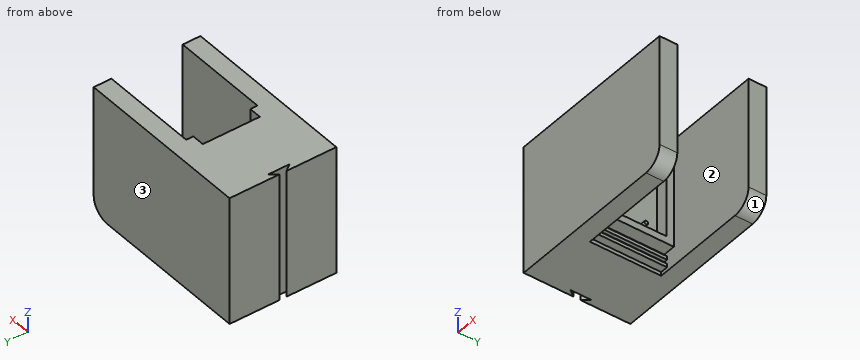
```python
from build123d import *

# Parameters (mm, degrees)
PAD_DEPTH       = 40.15
SKETCH001_W     = 72.15
SKETCH001_H     = 10
PAD001_DEPTH    = 100
FILLET_R        = 10
SKETCH002_W     = 57.4
SKETCH002_H     = 32.15
POCKET_DEPTH    = 7
SKETCH003_R     = 1.05
PAD002_DEPTH    = 3
POCKET001_DEPTH = 72.151


with BuildPart() as part:
    # Sketch → Pad (new body)
    with BuildSketch(Plane(origin=(24.695071, 0, 0), x_dir=(0, 0, 1), z_dir=(0, 1, 0))):
        Polygon((-27.089598, 5.251773), (34.310402, 5.251773), (34.310402, -39.748227), (-37.839598, -39.748227), (-37.839598, -4.048227), (-35.689598, -4.048227), (-35.689598, 0.251773), (-33.689598, 0.251773), (-33.689598, -1.748227), (-31.389598, -1.748227), (-31.389598, 0.251773), (-29.389598, 0.251773), (-29.389598, -1.748227), (-27.089598, -1.748227), align=None)
    extrude(amount=PAD_DEPTH)

    # Sketch001 (on Face4 of Pad) → Pad001 (join)
    with BuildSketch(Plane.ZY.offset(15.053156)):
        with Locations((-1.764598, -5)):
            Rectangle(SKETCH001_W, SKETCH001_H)
        with Locations((-1.764598, 45.15)):
            Rectangle(SKETCH001_W, SKETCH001_H)
    extrude(amount=-PAD001_DEPTH)

    # Fillet
    fillet_edges = [part.edges().sort_by_distance(p)[0] for p in [
        (84.946844, -5, -37.839598),
        (84.946844, 45.15, -37.839598),
    ]]
    fillet(fillet_edges, radius=FILLET_R)

    # Sketch002 (on Face6 of Fillet) → Pocket (cut)
    with BuildSketch(Plane(origin=(29.946844, 0, 0), x_dir=(0, 0, -1), z_dir=(1, 0, 0))):
        with Locations((-5.610402, 20.075)):
            Rectangle(SKETCH002_W, SKETCH002_H)
    extrude(amount=-POCKET_DEPTH, mode=Mode.SUBTRACT)

    # Sketch003 (on Face25 of Pocket) → Pad002 (join)
    with BuildSketch(Plane(origin=(22.946844, 0, 0), x_dir=(0, 0, -1), z_dir=(1, 0, 0))):
        with Locations((16.789598, 11.183873)):
            Circle(SKETCH003_R)
        with Locations((16.789598, 27.683873)):
            Circle(SKETCH003_R)
        with Locations((-7.210402, 11.183873)):
            Circle(SKETCH003_R)
    extrude(amount=PAD002_DEPTH)

    # Sketch004 (on Face20 of Pad002) → Pocket001 (cut, through all)
    with BuildSketch(Plane(origin=(24.695071, 0, -37.839598), x_dir=(-1, 0, 0), z_dir=(0, 0, -1))):
        Polygon((36.748227, 26.075), (39.748227, 22.075), (39.748227, 18.075), (36.748227, 14.075), align=None)
    extrude(amount=-POCKET001_DEPTH, mode=Mode.SUBTRACT)


solid = part.part
```
Verification items for the finished model (mm, model axes). Face numbers are marked on the shaded views. Coordinates: 2 decimals unless noted, no trailing zeros. Order: outer loops, then holes, each group sorted by start corner. A loop starts at its lowest first (then second) coordinate and runs counter-clockwise, first axis right, second up. Notation, with made-up numbers: (-6.5, 14) - (43.5, 14) arc R9 cw to (43.5, 20) - close; hole circle Ø3 at (88.5, 54). An arc over 180 degrees is marked (long way). Return JSON: item names as keys, results as strings.
(1) Section check A-A, the plane x = 42.5. Record the cut outline in (y, z).
Filled sheet:
{"outline": "(-10, -37.84) - (0, -37.84) - (0, 34.31) - (-10, 34.31) - close; (40.15, -37.84) - (50.15, -37.84) - (50.15, 34.31) - (40.15, 34.31) - close"}
(2) Mould release check, pull along Y, two halves, no side actions. Record for the marked faces 1, 2 and 3: pulls with the +Y half, pulls with the -Y half, needs draft (parallel to the pull), parting line crosses it, or undercut.
Filled sheet:
{"face 1": "needs draft", "face 2": "undercut", "face 3": "pulls with the +Y half"}
(3) Go/stop test with flat-tipped pins: pin 1 (5 mm diameter, centred on y = 34.5, z = 11.5, fed in from +X); pin 2 (1 mm diameter, centred on y = 18, z = -30.5, fed in from +X); pin 3 (5 mm diameter, centred on x = 33.5, y = 19.5, fed in from +Z); pin 4 (2.5 mm diameter, centred on y = 11.5, z = -37, fed in from +X). Record where each tip stops, or that it passes through.
Filled sheet:
{"pin 1": "stops at x = 29.95", "pin 2": "stops at x = 24.95", "pin 3": "passes through", "pin 4": "stops at x = 20.65"}
(4) Section check B-B, the plane z = -2.5. Record the cut outline in (x, y) (3 decimals).
Filled sheet:
{"outline": "(-15.053, -10) - (84.947, -10) - (84.947, 0) - (29.947, 0) - (29.947, 4) - (22.947, 4) - (22.947, 36.15) - (29.947, 36.15) - (29.947, 40.15) - (84.947, 40.15) - (84.947, 50.15) - (-15.053, 50.15) - (-15.053, 22.075) - (-12.053, 26.075) - (-12.053, 14.075) - (-15.053, 18.075) - close"}
(5) Section check C-C, the plane y = 8.5. Record the cut outline in (x, z).
Filled sheet:
{"outline": "(-15.05, -37.84) - (20.65, -37.84) - (20.65, -35.69) - (24.95, -35.69) - (24.95, -33.69) - (22.95, -33.69) - (22.95, -31.39) - (24.95, -31.39) - (24.95, -29.39) - (22.95, -29.39) - (22.95, -27.09) - (29.95, -27.09) - (29.95, -23.09) - (22.95, -23.09) - (22.95, 34.31) - (-15.05, 34.31) - close"}
(6) Thickness scan on line 1 along Y through (x, z) = (34, 4.5); line 2 along Y through (x, z) = (29.5, 9.5); line 3 along X through (y, z) = (8, 17.5). Record the ranges inside material, lowest first.
Filled sheet:
{"line 1": "y = -10 to 0, 40.15 to 50.15", "line 2": "y = -10 to 4, 36.15 to 50.15", "line 3": "x = -15.05 to 22.95"}
(7) Section check D-D, the plane z = -32.5. Record the cut outline in (x, y) (3 decimals).
Filled sheet:
{"outline": "(-15.053, -10) - (83.794, -10) - (83.794, 0) - (22.947, 0) - (22.947, 40.15) - (83.794, 40.15) - (83.794, 50.15) - (-15.053, 50.15) - (-15.053, 22.075) - (-12.053, 26.075) - (-12.053, 14.075) - (-15.053, 18.075) - close"}
